Geometry check sheet. Reference: the model listing, model coordinates, mm. Coordinates: 2 decimals unless noted, no trailing zeros. Order: outer loops, then holes, each group sorted by start corner. A loop starts at its lowest first (then second) coordinate and runs counter-clockwise, first axis right, second up. Notation, with made-up numbers: M -9,51.5 L 37,51.5 A7 ccw 37,61.5 Z; hole C 52,62 d3. An arc over 180 degrees is marked long. One line per item, written item: value. Start each with the question number.
1) Sectioned sample at D-D, the plane z = 57.15. Enter the section's corners in (x, y), then the cut area to 3 significant figures.
2) Sectioned sample at C-C, the plane x = 1.2. Enter the section's corners in (y, z).
3) Thickness scan on L1, parallel to Y at x = 0.6, z = 57.15; L2, parallel to Y at x = 0.75, z = 19.05; L3, parallel to Z at x = 0.8, y = 35. Record the ranges inside material, lowest first. Write a range as from..to.
4) Draft check along Z on faces 1 (the flat face through (1, 0, 38)), 2 (the flat face through (1, 25, 0)), 3 (the flat face through (1, 25, 76.2)), 4 (the cylindrical face through (0.852, 36.109, 12.223)). Enter one of: pulls with the +Z half, pulls with the -Z half, needs draft (parallel to the pull), parting line crosses it, or undercut.
5) Sectioned sample at A-A, the plane z = 19.05. Enter the section's corners in (x, y), then the cut area to 3 significant figures.
6) Sectioned sample at B-B, the plane y = 25.4. Enter the section's corners in (x, z).
```python
from build123d import *

# Parameters (mm, degrees)
SKETCH1_W           = 50.8
SKETCH1_H           = 76.2
BOSS_EXTRUDE1_DEPTH = 1.681219215
SKETCH3_R           = 11.1252
SKETCH3_R_2         = 12.7
CUT_EXTRUDE1_DEPTH  = 92.59643278


with BuildPart() as part:
    # Sketch1 → Boss-Extrude1 (new body)
    with BuildSketch(Plane.YZ):
        with Locations((25.4, 38.1)):
            Rectangle(SKETCH1_W, SKETCH1_H)
    extrude(amount=BOSS_EXTRUDE1_DEPTH)

    # Sketch3 → Cut-Extrude1 (cut, through all)
    with BuildSketch(Plane.YZ.offset(1.681219215)):
        with Locations(Location((25.4, 57.15, 0), (0, 0, 270))):
            Circle(SKETCH3_R)
        with Locations(Location((25.4, 19.05, 0), (0, 0, 270))):
            Circle(SKETCH3_R_2)
    extrude(amount=-CUT_EXTRUDE1_DEPTH, mode=Mode.SUBTRACT)


solid = part.part
```
Final values:
1. outline: M 0,0 L 1.68,0 L 1.68,14.27 L 0,14.27 Z; M 0,36.53 L 1.68,36.53 L 1.68,50.8 L 0,50.8 Z
1. area: 48.0 mm^2
2. outline: M 0,0 L 50.8,0 L 50.8,76.2 L 0,76.2 Z; hole C 25.4,19.05 d25.4; hole C 25.4,57.15 d22.25
3. L1: y = 0..14.27, 36.53..50.8
3. L2: y = 0..12.7, 38.1..50.8
3. L3: z = 0..10.74, 27.36..51.53, 62.77..76.2
4. face 1: needs draft
4. face 2: pulls with the -Z half
4. face 3: pulls with the +Z half
4. face 4: undercut
5. outline: M 0,0 L 1.68,0 L 1.68,12.7 L 0,12.7 Z; M 0,38.1 L 1.68,38.1 L 1.68,50.8 L 0,50.8 Z
5. area: 42.7 mm^2
6. outline: M 0,0 L 1.68,0 L 1.68,6.35 L 0,6.35 Z; M 0,31.75 L 1.68,31.75 L 1.68,46.02 L 0,46.02 Z; M 0,68.28 L 1.68,68.28 L 1.68,76.2 L 0,76.2 Z
